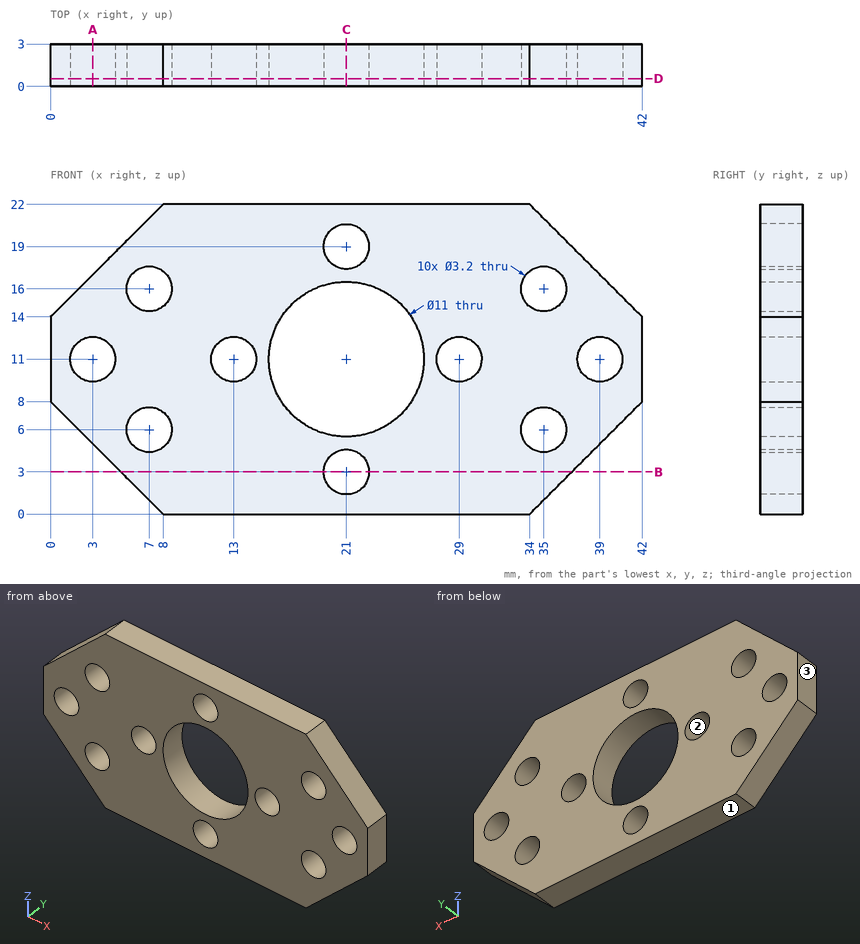
Design review of the part shown in the three views and the two pictorial views. Dimensions are in mm from the part's minimum x, y and z. Round coordinates to 2 decimals unless told otherwise and drop trailing zeros. Loops run counter-clockwise (first coordinate to the right, second up) from the corner with the lowest first, then second, coordinate; pieces in that order, holes last. Notation, with made-up numbers: M -26,-7.75 L -19,-7.75 A31 ccw -19,30.25 Z; hole C 72,39.5 d3. An arc over 180 degrees is marked long. Put each result on its own line as item: value.
Q1. Consider section A-A, the plane x = 3. Give the boundary of the cut face in (y, z), then the cut area to 3 significant figures.
Result set:
outline: M 0,5 L 3,5 L 3,9.4 L 0,9.4 Z; M 0,12.6 L 3,12.6 L 3,17 L 0,17 Z
area: 26.4 mm²
Q2. Consider section B-B, the plane z = 3. Give the boundary of the cut face in (x, y), then the cut area to 3 significant figures.
Result set:
outline: M 5,0 L 19.4,0 L 19.4,3 L 5,3 Z; M 22.6,0 L 37,0 L 37,3 L 22.6,3 Z
area: 86.4 mm²
Q3. Consider section D-D, the plane y = 0.55. Count the separate pieces of the cut face and the enclosed holes in it, then the cut area to 3 significant figures.
Result set:
separate pieces: 1
enclosed holes: 11
area: 621 mm²
Q4. Mouldability with a two-part tool opening along Z and no side actions: class the marked faces 1, 2 and 3 as released by +Z, released by -Z, zero draft, split by the parting line, or undercut.
Result set:
face 1: released by -Z
face 2: undercut
face 3: zero draft
Q5. For pin 1 (6.5 mm diameter, centred on x = 21, z = 11, fed in from +Y); pin 2 (1.5 mm diameter, centred on y = 0.5, z = 17, fed in from +X), all flat-tipped, find the tip position at first contact; note any pin that passes through.
Result set:
pin 1: passes through
pin 2: stops at x = 39.75
Q6. To check wall thickness, follow L1, parallel to X at y = 1.8, z = 11; L2, parallel to Z at x = 6, y = 1.7; L3, parallel to X at y = 2.05, z = 7.25. State the ranges of each line that lie inside material, in increasing order.
Result set:
L1: x = 0 to 1.4, 4.6 to 11.4, 14.6 to 15.5, 26.5 to 27.4, 30.6 to 37.4, 40.6 to 42
L2: z = 2 to 4.75, 7.25 to 14.75, 17.25 to 20
L3: x = 0.75 to 6, 8 to 16.98, 25.02 to 34, 36 to 41.25
Q7. Consider section C-C, the plane x = 21. Give the boundary of the cut face in (y, z), then the cut area to 3 significant figures.
Result set:
outline: M 0,0 L 3,0 L 3,1.4 L 0,1.4 Z; M 0,4.6 L 3,4.6 L 3,5.5 L 0,5.5 Z; M 0,16.5 L 3,16.5 L 3,17.4 L 0,17.4 Z; M 0,20.6 L 3,20.6 L 3,22 L 0,22 Z
area: 13.8 mm²
